from build123d import *

# Parameters (mm, degrees)
SKETCH125_W     = 108
SKETCH125_H     = 108
PAD050_DEPTH    = 2
FILLET009_R     = 8
SKETCH126_R     = 3.25
POCKET049_DEPTH = 1
POCKET048_DEPTH = 2.001


with BuildPart() as part:
    # Sketch125 → Pad050 (new body)
    with BuildSketch(Plane.XY):
        with Locations((54, 54)):
            Rectangle(SKETCH125_W, SKETCH125_H)
    extrude(amount=PAD050_DEPTH)

    # Fillet009
    fillet009_edges = [part.edges().sort_by_distance(p)[0] for p in [
        (108, 0, 1),
        (108, 108, 1),
        (0, 108, 1),
        (0, 0, 1),
    ]]
    fillet(fillet009_edges, radius=FILLET009_R)

    # Sketch126 (on Face5 of Fillet009) → Pocket049 (cut)
    with BuildSketch(Plane.XY.offset(2)):
        with Locations((8, 8)):
            Circle(SKETCH126_R)
        with Locations((100, 8)):
            Circle(SKETCH126_R)
        with Locations((100, 100)):
            Circle(SKETCH126_R)
        with Locations((8, 100)):
            Circle(SKETCH126_R)
    extrude(amount=-POCKET049_DEPTH, mode=Mode.SUBTRACT)

    # Sketch127 (on Face5 of Pocket049) → Pocket048 (cut, through all)
    with BuildSketch(Plane.XY.offset(2)):
        with BuildLine():
            Line((2, 94.708497), (2, 13.291503))
            ThreePointArc((13.291503, 2), (13.655204, 13.655204), (2, 13.291503))
            Line((13.291503, 2), (94.708497, 2))
            ThreePointArc((106, 13.291503), (94.343146, 13.656854), (94.708497, 2))
            Line((106, 94.708497), (106, 13.291503))
            ThreePointArc((94.708497, 106), (94.342737, 94.342737), (106, 94.708497))
            Line((13.291503, 106), (94.708497, 106))
            ThreePointArc((2, 94.708497), (13.656854, 94.343146), (13.291503, 106))
        make_face()
    extrude(amount=-POCKET048_DEPTH, mode=Mode.SUBTRACT)


with BuildPart() as part_1:
    # Body022 placement: moved
    add(part.part.moved(Location((0, 0, 184))))


solid = part_1.part
Geometry check sheet. Reference: the model listing, model coordinates, mm. A direction names the side the tool comes from. Give positions to 0.01 mm unless a question says otherwise; leave off trailing zeros. Write each loop counter-clockwise with the first axis right and the second up, starting at its lowest first coordinate (ties: lowest second). Pieces come first, ordered by that corner, then holes.
1) Cross-section at D-D (x = 10). Record the boundary of the cut face in (y, z).
Values follow:
outline: (0, 184) - (15.74, 184) - (15.74, 186) - (10.56, 186) - (10.56, 185) - (5.44, 185) - (5.44, 186) - (0, 186) - close; (92.25, 184) - (108, 184) - (108, 186) - (102.56, 186) - (102.56, 185) - (97.44, 185) - (97.44, 186) - (92.25, 186) - close
2) Cross-section at C-C (z = 184.6). Record the boundary of the cut face in (x, y).
Values follow:
outline: (0, 8) arc R8 ccw to (8, 0) - (100, 0) arc R8 ccw to (108, 8) - (108, 100) arc R8 ccw to (100, 108) - (8, 108) arc R8 ccw to (0, 100) - close; hole (2, 13.29) arc R8 cw (long way) to (13.29, 2) - (94.71, 2) arc R8 cw (long way) to (106, 13.29) - (106, 94.71) arc R8 cw (long way) to (94.71, 106) - (13.29, 106) arc R8 cw (long way) to (2, 94.71) - close
3) Go/stop test with a flat-tipped pin: pin 1 Ø2 at (x, y) = (99.5, 100) entering from +Z. Record where the tip stops, or that it passes through.
Values follow:
pin 1: stops at z = 185
4) Set-up check for faces 4 (the face through (2.281, 2.406, 185.014)), 5 (the face through (5.605, 10.197, 185.507)): record each of +Z, -Z, +X, -X, +Y, -Y from which the full face is reachable in a straight line by a thin tool's end or side.
Values follow:
face 4: +Z, -Z, -X, -Y
face 5: +Z
5) Thickness scan on line 1 (Y direction, x = 8, z = 185.75); line 2 (X direction, y = 81.5, z = 185.25). Record the ranges inside material, lowest first.
Values follow:
line 1: y = 0 to 4.75, 11.25 to 16, 92 to 96.75, 103.25 to 108
line 2: x = 0 to 2, 106 to 108
6) Cross-section at A-A (y = 47.5). Record the boundary of the cut face in (x, z).
Values follow:
outline: (0, 184) - (2, 184) - (2, 186) - (0, 186) - close; (106, 184) - (108, 184) - (108, 186) - (106, 186) - close
7) Release check for a two-part mould opening along X. For faces 1 (the face through (8, 100, 185)), 2 (the face through (37.7, 106.3, 186)), 3 (the face through (105.719, 105.594, 185.014)) record: released by +X, released by -X, zero draft, split by the parting line, or undercut.
Values follow:
face 1: undercut
face 2: zero draft
face 3: released by +X
